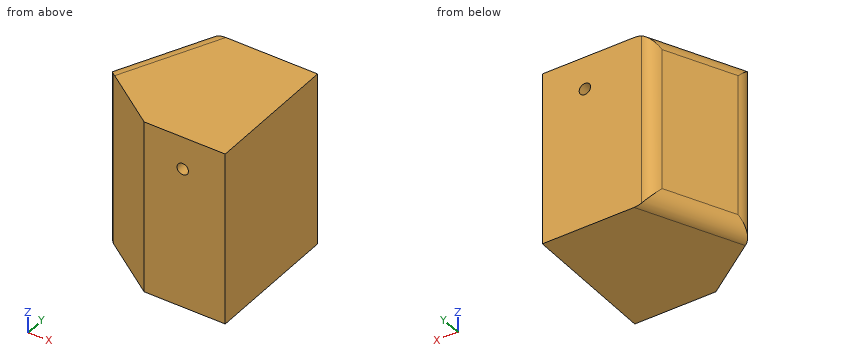
from build123d import *

# Parameters (mm, degrees)
F1_DEPTH = 96.519992
F2_R     = 8.781853
F4_D     = 6.35


with BuildPart() as f1:
    # F0 (on Top) → F1 (new body)
    with BuildSketch(Plane.XY):
        Polygon((-23.089193, 0), (15.667696, -27.583569), (60.70821, -27.583569), (60.70821, 48.24049), (0, 48.24049), align=None)
    extrude(amount=F1_DEPTH)

    # F2
    f2_edges = [f1.edges().sort_by_distance(p)[0] for p in [
        (0, 48.24049, 48.259996),
        (-23.089193, 0, 48.259996),
        (-11.544596, 24.120245, 0),
        (-11.544596, 24.120245, 96.519992),
    ]]
    fillet(f2_edges, radius=F2_R)

    # F4 (through all)
    with Locations(Plane.XZ.offset(27.583569)):
        with Locations((37.103444, 78.396708)):
            Hole(F4_D / 2)


solid = f1.part
CAD build for the part. Positions are in the model's coordinates, mm. Give positions to 0.01 mm unless a question says otherwise; leave off trailing zeros. Order: outer loops, then holes, each group sorted by start corner. A loop starts at its lowest first (then second) coordinate and runs counter-clockwise, first axis right, second up. Notation, with made-up numbers: (-15, 62.5) - (23, 62.5) arc R23 cw to (23, 98.5) - close; hole circle Ø4 at (-17, 6). An arc over 180 degrees is marked (long way). Write each question's results on one line, items separated by ' | '.
1. Probe L1, parallel to Z at x = 38, y = -8; L2, parallel to X at y = 29, z = 56; L3, parallel to X at y = 9.5, z = 85. List the from-to ranges inside material, lowest first. Write a range as from..to.
Calculated:
L1: z = 0..75.35, 81.44..96.52 | L2: x = -9.21..60.71 | L3: x = -18.54..60.71
2. Pin check, flat tips, straight feed: pin 1 (1 mm diameter, centred on x = 45, y = -8.5, fed in from -Z); pin 2 (5.5 mm diameter, centred on x = 37.1, z = 78.4, fed in from -Y); pin 3 (12 mm diameter, centred on y = -16.5, z = 81.5, fed in from -X); pin 4 (8 mm diameter, centred on x = -9, z = 66, fed in from +Y). Stop position of each tip, or through.
Calculated:
pin 1: stops at z = 0 | pin 2: passes through | pin 3: stops at x = -8.34 | pin 4: stops at y = 37.79
3. Saw through at A-A on x = 37. List the corners of the cut face in (y, z).
Calculated:
outline: (-27.58, 0) - (48.24, 0) - (48.24, 75.22) - (-27.58, 75.22) - close; (-27.58, 81.57) - (48.24, 81.57) - (48.24, 96.52) - (-27.58, 96.52) - close
4. Saw through at B-B on z = 36.5. List the corners of the cut face in (x, y).
Calculated:
outline: (-19.9, 6.66) arc R8.78 ccw to (-17.07, -4.28) - (15.67, -27.58) - (60.71, -27.58) - (60.71, 48.24) - (5.53, 48.24) arc R8.78 ccw to (-2.39, 43.25) - close
5. Saw through at D-D on y = -6.5. List the corners of the cut face in (x, z) (3 decimals).
Calculated:
outline: (-13.956, 0) - (60.708, 0) - (60.708, 96.52) - (-13.956, 96.52) - close; hole circle Ø6.35 at (37.103, 78.397)
6. Saw through at C-C on y = -21. List the corners of the cut face in (x, z) (3 decimals), and give its area (3 significant figures).
Calculated:
outline: (6.417, 0) - (60.708, 0) - (60.708, 96.52) - (6.417, 96.52) - close; hole circle Ø6.35 at (37.103, 78.397) | area: 5,210 mm2
